Part model, mm, in its own coordinate system. A direction names the side the tool comes from. Round coordinates to 2 decimals unless told otherwise and drop trailing zeros. Order: outer loops, then holes, each group sorted by start corner. A loop starts at its lowest first (then second) coordinate and runs counter-clockwise, first axis right, second up. Notation, with made-up numbers: (89, 76.25) - (143, 76.25) arc R7 cw to (143, 80.25) - close; hole circle Ø1 at (-28.5, 67.25). An arc over 180 degrees is marked (long way). Answer as a JSON object with one key per item and string values.
```python
from build123d import *

# Parameters (mm, degrees)
SKETCH1_W           = 100
SKETCH1_H           = 156
SKETCH1_R           = 7
SKETCH1_R_2         = 4
SKETCH1_R_3         = 3.6
BOSS_EXTRUDE1_DEPTH = 14
FILLET1_R           = 5
SKETCH1_3_R         = 7
SKETCH1_3_R_2       = 3.6
CUT_EXTRUDE1_DEPTH  = 8


with BuildPart() as part:
    # Sketch1 → Boss-Extrude1 (new body)
    # profile 1 of 3: a face of its own
    with BuildSketch(Plane(origin=(0, 0, 0), x_dir=(0, 0, -1), z_dir=(1, 0, 0))):
        with Locations((50, 78)):
            Rectangle(SKETCH1_W, SKETCH1_H)
        with Locations((50, 40)):
            Circle(SKETCH1_R, mode=Mode.SUBTRACT)
        with Locations((50, 116)):
            Circle(SKETCH1_R, mode=Mode.SUBTRACT)
        with Locations((90, 78)):
            Circle(SKETCH1_R_2, mode=Mode.SUBTRACT)
        with Locations((10, 78)):
            Circle(SKETCH1_R_2, mode=Mode.SUBTRACT)
    # profile 2 of 3: a face of its own
    with BuildSketch(Plane(origin=(0, 0, 0), x_dir=(0, 0, -1), z_dir=(1, 0, 0))):
        with Locations((50, 40)):
            Circle(SKETCH1_R)
        with Locations((50, 40)):
            Circle(SKETCH1_R_3, mode=Mode.SUBTRACT)
    # profile 3 of 3: a face of its own
    with BuildSketch(Plane(origin=(0, 0, 0), x_dir=(0, 0, -1), z_dir=(1, 0, 0))):
        with Locations((50, 116)):
            Circle(SKETCH1_R)
        with Locations((50, 116)):
            Circle(SKETCH1_R_3, mode=Mode.SUBTRACT)
    extrude(amount=BOSS_EXTRUDE1_DEPTH)

    # Fillet1
    fillet1_edges = [part.edges().sort_by_distance(p)[0] for p in [
        (7, 0, 0),
        (7, 156, 0),
        (7, 156, -100),
        (7, 0, -100),
    ]]
    fillet(fillet1_edges, radius=FILLET1_R)

    # Sketch1_3 → Cut-Extrude1 (cut)
    # profile 1 of 2: a face of its own
    with BuildSketch(Plane(origin=(0, 0, 0), x_dir=(0, 0, -1), z_dir=(1, 0, 0))):
        with Locations((50, 116)):
            Circle(SKETCH1_3_R)
        with Locations((50, 116)):
            Circle(SKETCH1_3_R_2, mode=Mode.SUBTRACT)
    # profile 2 of 2: a face of its own
    with BuildSketch(Plane(origin=(0, 0, 0), x_dir=(0, 0, -1), z_dir=(1, 0, 0))):
        with Locations((50, 40)):
            Circle(SKETCH1_3_R)
        with Locations((50, 40)):
            Circle(SKETCH1_3_R_2, mode=Mode.SUBTRACT)
    extrude(amount=CUT_EXTRUDE1_DEPTH, mode=Mode.SUBTRACT)


solid = part.part
```
Item 1: Cut at A-A (y = 78). Write the cut outline in (x, z).
Taken from the geometry:
{"outline": "(0, -100) - (14, -100) - (14, -94) - (0, -94) - close; (0, -86) - (14, -86) - (14, -14) - (0, -14) - close; (0, -6) - (14, -6) - (14, 0) - (0, 0) - close"}
Item 2: Cut at C-C (x = 4.5). Write the cut outline in (y, z), plus the area to 3 significant figures.
Taken from the geometry:
{"outline": "(0, -95) arc R5 ccw to (5, -100) - (151, -100) arc R5 ccw to (156, -95) - (156, -5) arc R5 ccw to (151, 0) - (5, 0) arc R5 ccw to (0, -5) - close; hole circle Ø14 at (40, -50); hole circle Ø8 at (78, -90); hole circle Ø8 at (78, -10); hole circle Ø14 at (116, -50)", "area": "15,200 mm2"}
Item 3: Cut at D-D (y = 116). Write the cut outline in (x, z).
Taken from the geometry:
{"outline": "(0, -100) - (14, -100) - (14, -53.6) - (8, -53.6) - (8, -57) - (0, -57) - close; (0, -43) - (8, -43) - (8, -46.4) - (14, -46.4) - (14, 0) - (0, 0) - close"}
Item 4: Cut at B-B (z = -90). Write the cut outline in (x, y), plus the area to 3 significant figures.
Taken from the geometry:
{"outline": "(0, 0) - (14, 0) - (14, 74) - (0, 74) - close; (0, 82) - (14, 82) - (14, 156) - (0, 156) - close", "area": "2,070 mm2"}
Item 5: Probe L1, parallel to Y at x = 6.25, z = -50; L2, parallel to Y at x = 11.3, z = -50; L3, parallel to Z at x = 13.25, y = 81. List the from-to ranges inside material, lowest first. Write a range as from..to.
Taken from the geometry:
{"L1": "0..33, 47..109, 123..156", "L2": "0..36.4, 43.6..112.4, 119.6..156", "L3": "-100..-92.65, -87.35..-12.65, -7.35..0"}
Item 6: Tool access for faces 4 (the flat face through (7, 0, -49)), 5 (the flat face through (8, 37, -53)): list every direction of +Z, -Z, +X, -X, +Y, -Y with a clear straight run to the whole face (end or side of a thin tool).
Taken from the geometry:
{"face 4": "+Z, -Z, +X, -X, -Y", "face 5": "-X"}
Item 7: Drop flat-ended pins along their axis: P1, Ø6.5, axis at y = 78, z = -90, coming from the -X side; P2, Ø7, axis at y = 40.5, z = -51, coming from the -X side. Give the stop position or say it passes through.
Taken from the geometry:
{"P1": "through", "P2": "x = 8"}
Item 8: Two-plate mould, pull along Y, no slides. Class faces 1 (the cylindrical face through (7, 1, -98)), 2 (the cylindrical face through (10.958, 117.081, -53.434)), 3 (the flat face through (7, 77, 0)): pulls with the +Y half, pulls with the -Y half, needs draft (parallel to the pull), parting line crosses it, or undercut.
Taken from the geometry:
{"face 1": "pulls with the -Y half", "face 2": "undercut", "face 3": "needs draft"}
